from build123d import *

# Parameters (mm, degrees)
EXTRUDE_1_DEPTH     = 2.5
SKETCH_1_5_R        = 0.75
EXTRUDE_3_DEPTH     = 1.5
SKETCH_1_6_W        = 13.2
SKETCH_1_6_H        = 2.5
EXTRUDE_4_DEPTH     = 3
SKETCH_1_7_W        = 2.5
SKETCH_1_7_H        = 14
EXTRUDE_5_DEPTH     = 5.5
SKETCH_1_8_W        = 7.2
SKETCH_1_8_H        = 2.5
SKETCH_1_8_W_2      = 2.5
SKETCH_1_8_H_2      = 5
EXTRUDE_6_DEPTH     = 20.5
CUT_EXTRUDE_START   = -1.4
SKETCH_1_9_R        = 0.75
CUT_EXTRUDE_1_DEPTH = 1.4


with BuildPart() as part:
    # Sketch 1 → Extrude 1 (new body)
    with BuildSketch(Plane.XY):
        with BuildLine():
            Line((-26.5, 39.5), (26.5, 39.5))
            ThreePointArc((26.5, 39.5), (28.621320344, 38.621320344), (29.5, 36.5))
            Line((29.5, 36.5), (29.5, -36.5))
            ThreePointArc((29.5, -36.5), (28.621320344, -38.621320344), (26.5, -39.5))
            Line((26.5, -39.5), (-26.5, -39.5))
            ThreePointArc((-26.5, -39.5), (-28.621320344, -38.621320344), (-29.5, -36.5))
            Line((-29.5, -36.5), (-29.5, 36.5))
            ThreePointArc((-29.5, 36.5), (-28.621320344, 38.621320344), (-26.5, 39.5))
        make_face()
    extrude(amount=-EXTRUDE_1_DEPTH)

    # Sketch 1_5 → Extrude 3 (add)
    # profile 1 of 4: a face of its own
    with BuildSketch(Plane.XY):
        with BuildLine():
            Line((-21, 31.5), (-21, 37))
            Line((-21, 37), (-24, 37))
            ThreePointArc((-24, 37), (-26.121320344, 36.121320344), (-27, 34))
            Line((-27, 34), (-27, 29.5))
            Line((-27, 29.5), (-23, 29.5))
            ThreePointArc((-23, 29.5), (-21.585786438, 30.085786438), (-21, 31.5))
        make_face()
        with Locations((-23, 31.5)):
            Circle(SKETCH_1_5_R, mode=Mode.SUBTRACT)
    # profile 2 of 4: a face of its own
    with BuildSketch(Plane.XY):
        with BuildLine():
            Line((27, -34), (27, -32.5))
            Line((27, -32.5), (23, -32.5))
            ThreePointArc((23, -32.5), (21.585786438, -33.085786438), (21, -34.5))
            Line((21, -34.5), (21, -37))
            Line((21, -37), (24, -37))
            ThreePointArc((24, -37), (26.121320344, -36.121320344), (27, -34))
        make_face()
        with Locations((23, -34.5)):
            Circle(SKETCH_1_5_R, mode=Mode.SUBTRACT)
    # profile 3 of 4: a face of its own
    with BuildSketch(Plane.XY):
        with BuildLine():
            Line((-23, -32.5), (-27, -32.5))
            Line((-27, -32.5), (-27, -34))
            ThreePointArc((-27, -34), (-26.121320344, -36.121320344), (-24, -37))
            Line((-24, -37), (-21.7, -37))
            Line((-21.7, -37), (-21, -37))
            Line((-21, -37), (-21, -34.5))
            ThreePointArc((-21, -34.5), (-21.585786438, -33.085786438), (-23, -32.5))
        make_face()
        with Locations((-23, -34.5)):
            Circle(SKETCH_1_5_R, mode=Mode.SUBTRACT)
    # profile 4 of 4: a face of its own
    with BuildSketch(Plane.XY):
        with BuildLine():
            Line((24, 37), (21, 37))
            Line((21, 37), (21, 31.5))
            ThreePointArc((21, 31.5), (21.585786438, 30.085786438), (23, 29.5))
            Line((23, 29.5), (27, 29.5))
            Line((27, 29.5), (27, 34))
            ThreePointArc((27, 34), (26.121320344, 36.121320344), (24, 37))
        make_face()
        with Locations((23, 31.5)):
            Circle(SKETCH_1_5_R, mode=Mode.SUBTRACT)
    extrude(amount=EXTRUDE_3_DEPTH)

    # Sketch 1_6 → Extrude 4 (add)
    with BuildSketch(Plane.XY):
        with Locations((-7.9, 38.25)):
            Rectangle(SKETCH_1_6_W, SKETCH_1_6_H)
        with Locations((12.5, 38.25)):
            Rectangle(SKETCH_1_6_W, SKETCH_1_6_H)
        Polygon((-21.7, -37), (-21.7, -39.5), (-0.1, -39.5), (-0.1, -37), (-21, -37), align=None)
    extrude(amount=EXTRUDE_4_DEPTH)

    # Sketch 1_7 → Extrude 5 (add)
    with BuildSketch(Plane.XY):
        with Locations((-28.25, 14)):
            Rectangle(SKETCH_1_7_W, SKETCH_1_7_H)
        with Locations((-28.25, -5)):
            Rectangle(SKETCH_1_7_W, SKETCH_1_7_H)
    extrude(amount=EXTRUDE_5_DEPTH)

    # Sketch 1_8 → Extrude 6 (add)
    with BuildSketch(Plane.XY):
        with BuildLine():
            Line((26.5, 39.5), (19.1, 39.5))
            Line((19.1, 39.5), (19.1, 37))
            Line((19.1, 37), (21, 37))
            Line((21, 37), (24, 37))
            ThreePointArc((24, 37), (26.121320344, 36.121320344), (27, 34))
            Line((27, 34), (27, 29.5))
            Line((27, 29.5), (27, -32.5))
            Line((27, -32.5), (27, -34))
            ThreePointArc((27, -34), (26.121320344, -36.121320344), (24, -37))
            Line((24, -37), (21, -37))
            Line((21, -37), (-0.1, -37))
            Line((-0.1, -37), (-0.1, -39.5))
            Line((-0.1, -39.5), (26.5, -39.5))
            ThreePointArc((26.5, -39.5), (28.621320344, -38.621320344), (29.5, -36.5))
            Line((29.5, -36.5), (29.5, 36.5))
            ThreePointArc((29.5, 36.5), (28.621320344, 38.621320344), (26.5, 39.5))
        make_face()
        with Locations((2.3, 38.25)):
            Rectangle(SKETCH_1_8_W, SKETCH_1_8_H)
        with BuildLine():
            Line((-14.5, 39.5), (-26.5, 39.5))
            ThreePointArc((-26.5, 39.5), (-28.621320344, 38.621320344), (-29.5, 36.5))
            Line((-29.5, 36.5), (-29.5, 21))
            Line((-29.5, 21), (-27, 21))
            Line((-27, 21), (-27, 29.5))
            Line((-27, 29.5), (-27, 34))
            ThreePointArc((-27, 34), (-26.121320344, 36.121320344), (-24, 37))
            Line((-24, 37), (-21, 37))
            Line((-21, 37), (-14.5, 37))
            Line((-14.5, 37), (-14.5, 39.5))
        make_face()
        with Locations((-28.25, 4.5)):
            Rectangle(SKETCH_1_8_W_2, SKETCH_1_8_H_2)
        with BuildLine():
            Line((-27, -12), (-29.5, -12))
            Line((-29.5, -12), (-29.5, -36.5))
            ThreePointArc((-29.5, -36.5), (-28.621320344, -38.621320344), (-26.5, -39.5))
            Line((-26.5, -39.5), (-21.7, -39.5))
            Line((-21.7, -39.5), (-21.7, -37))
            Line((-21.7, -37), (-24, -37))
            ThreePointArc((-24, -37), (-26.121320344, -36.121320344), (-27, -34))
            Line((-27, -34), (-27, -32.5))
            Line((-27, -32.5), (-27, -12))
        make_face()
    extrude(amount=EXTRUDE_6_DEPTH)

    # Sketch 1_9 → Cut-Extrude 1 (cut)
    with BuildSketch(Plane.XY.offset(CUT_EXTRUDE_START)):
        with Locations((-23, 31.5)):
            Circle(SKETCH_1_9_R)
        with Locations((23, 31.5)):
            Circle(SKETCH_1_9_R)
        with Locations((23, -34.5)):
            Circle(SKETCH_1_9_R)
        with Locations((-23, -34.5)):
            Circle(SKETCH_1_9_R)
    extrude(amount=CUT_EXTRUDE_1_DEPTH, mode=Mode.SUBTRACT)


solid = part.part
Read the model definition and answer for the solid it produces. Units are mm, in the model's axes. A direction names the side the tool comes from. Round coordinates to 2 decimals unless told otherwise and drop trailing zeros. Write each loop counter-clockwise with the first axis right and the second up, starting at its lowest first coordinate (ties: lowest second). Pieces come first, ordered by that corner, then holes. Notation, with made-up numbers: (12.25, -31.5) - (45.25, -31.5) arc R17 ccw to (45.25, -2.5) - close; hole circle Ø5 at (46.25, 69). An arc over 180 degrees is marked (long way). Use a Markdown table: item, result.
(1) Each of these flat-tipped pins is pushed along its axis until it touches: pin 1 Ø0.8 at (x, y) = (-23, -34.5) entering from +Z; pin 2 Ø1 at (y, z) = (0.5, 11.5) entering from -X; pin 3 Ø1.2 at (x, y) = (-8.5, 39) entering from +Z. Where does it stop, or does it pass through?
Reported:
| item | result |
|---|---|
| pin 1 | z = -1.4 |
| pin 2 | x = 27 |
| pin 3 | z = 3 |
(2) The part is cut by section C-C (z = 13.75). State how many separate pieces and enclosed holes the cut face has, then the cut area to 3 significant figures.
Reported:
| item | result |
|---|---|
| separate pieces | 5 |
| enclosed holes | 0 |
| area | 475 mm2 |
(3) Which of the six approach directions +Z, -Z, +X, -X, +Y, -Y give full straight-line access (tool end or side, diameter ignored) to faces 5 (the flat face through (-28, 21, 13)), 6 (the flat face through (0, 37, 10)), 7 (the flat face through (-11, -38, 3)), 8 (the flat face through (-1.3, 38, 12))?
Reported:
| item | result |
|---|---|
| face 5 | +Z, -X |
| face 6 | +Z |
| face 7 | +Z, -Y |
| face 8 | +Z, +Y, -Y |
(4) Straight lines are drawn through the part: line 1 along X through (y, z) = (-34.5, -0.1); line 2 along Y through (x, z) = (-23, -0.65); line 3 along Y through (x, z) = (23, 0.8). For each, find the intervals that lie inside material, in ascending order. Write a range as [from, to].
Reported:
| item | result |
|---|---|
| line 1 | [-29.5, -23.75], [-22.25, 22.25], [23.75, 29.5] |
| line 2 | [-39.5, -35.25], [-33.75, 30.75], [32.25, 39.5] |
| line 3 | [-39.5, -35.25], [-33.75, -32.5], [29.5, 30.75], [32.25, 39.5] |
(5) The part is cut by section A-A (y = -15.5). Write down the section's boundary in (x, z).
Reported:
| item | result |
|---|---|
| outline | (-29.5, -2.5) - (29.5, -2.5) - (29.5, 20.5) - (27, 20.5) - (27, 0) - (-27, 0) - (-27, 20.5) - (-29.5, 20.5) - close |
(6) The part is cut by section B-B (x = -3.5). Write down the section's boundary in (y, z).
Reported:
| item | result |
|---|---|
| outline | (-39.5, -2.5) - (39.5, -2.5) - (39.5, 3) - (37, 3) - (37, 0) - (-37, 0) - (-37, 3) - (-39.5, 3) - close |
(7) The mould has two halves that part along Y. Classify faces 1 (the flat face through (6, -39.5, 6)), 2 (the flat face through (0, 39.5, 6)), 3 (the cylindrical face through (21.57, 30.1, 0.74)), 4 (the flat face through (-21.7, -38, 12)): released by +Y, released by -Y, zero draft, split by the parting line, or undercut.
Reported:
| item | result |
|---|---|
| face 1 | released by -Y |
| face 2 | released by +Y |
| face 3 | undercut |
| face 4 | zero draft |
